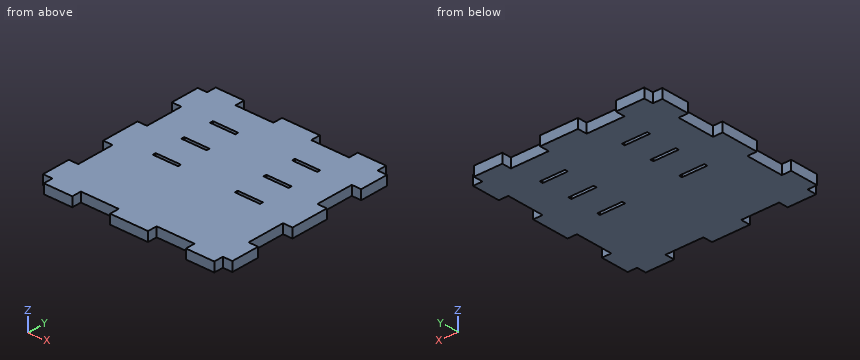
```python
from build123d import *

# Parameters (mm, degrees)
SKETCH1_W           = 190.5
SKETCH1_H           = 190.5
BOSS_EXTRUDE2_DEPTH = 9.525
SKETCH2_W           = 38.1
SKETCH2_H           = 9.525
CUT_EXTRUDE1_DEPTH  = 9.525
SKETCH3_W           = 38.1
SKETCH3_H           = 9.525
CUT_EXTRUDE2_DEPTH  = 9.525
SKETCH4_W           = 9.525
SKETCH4_H           = 38.1
CUT_EXTRUDE3_DEPTH  = 9.525
SKETCH5_W           = 9.525
SKETCH5_H           = 38.1
CUT_EXTRUDE4_DEPTH  = 9.525
SKETCH6_W           = 38.1
SKETCH6_H           = 9.525
CUT_EXTRUDE5_DEPTH  = 9.525
SKETCH7_W           = 38.1
SKETCH7_H           = 9.525
CUT_EXTRUDE6_DEPTH  = 9.525
SKETCH8_W           = 9.525
SKETCH8_H           = 38.1
CUT_EXTRUDE7_DEPTH  = 9.525
SKETCH9_W           = 9.525
SKETCH9_H           = 38.1
CUT_EXTRUDE8_DEPTH  = 9.525
SKETCH10_W          = 9.525
SKETCH10_H          = 9.525
CUT_EXTRUDE9_DEPTH  = 9.525
SKETCH11_W          = 9.525
SKETCH11_H          = 9.525
CUT_EXTRUDE10_DEPTH = 9.525
SKETCH12_W          = 9.525
SKETCH12_H          = 9.525
CUT_EXTRUDE11_DEPTH = 9.525
SKETCH13_W          = 9.525
SKETCH13_H          = 9.525
CUT_EXTRUDE12_DEPTH = 9.525
SKETCH14_W          = 25.4
SKETCH14_H          = 3.175
CUT_EXTRUDE13_DEPTH = 204.230898008


with BuildPart() as part:
    # Sketch1 → Boss-Extrude2 (new body)
    with BuildSketch(Plane.XY):
        with Locations((26.090217391, -67.50326087)):
            Rectangle(SKETCH1_W, SKETCH1_H)
    extrude(amount=BOSS_EXTRUDE2_DEPTH)

    # Sketch2 → Cut-Extrude1 (cut)
    with BuildSketch(Plane.XY.offset(9.525)):
        with Locations((-12.009782609, 22.98423913)):
            Rectangle(SKETCH2_W, SKETCH2_H)
    extrude(amount=-CUT_EXTRUDE1_DEPTH, mode=Mode.SUBTRACT)

    # Sketch3 → Cut-Extrude2 (cut)
    with BuildSketch(Plane.XY.offset(9.525)):
        with Locations((64.190217391, 22.98423913)):
            Rectangle(SKETCH3_W, SKETCH3_H)
    extrude(amount=-CUT_EXTRUDE2_DEPTH, mode=Mode.SUBTRACT)

    # Sketch4 → Cut-Extrude3 (cut)
    with BuildSketch(Plane.XY.offset(9.525)):
        with Locations((116.577717391, -29.40326087)):
            Rectangle(SKETCH4_W, SKETCH4_H)
    extrude(amount=-CUT_EXTRUDE3_DEPTH, mode=Mode.SUBTRACT)

    # Sketch5 → Cut-Extrude4 (cut)
    with BuildSketch(Plane.XY.offset(9.525)):
        with Locations((116.577717391, -105.60326087)):
            Rectangle(SKETCH5_W, SKETCH5_H)
    extrude(amount=-CUT_EXTRUDE4_DEPTH, mode=Mode.SUBTRACT)

    # Sketch6 → Cut-Extrude5 (cut)
    with BuildSketch(Plane.XY.offset(9.525)):
        with Locations((64.190217391, -157.99076087)):
            Rectangle(SKETCH6_W, SKETCH6_H)
    extrude(amount=-CUT_EXTRUDE5_DEPTH, mode=Mode.SUBTRACT)

    # Sketch7 → Cut-Extrude6 (cut)
    with BuildSketch(Plane.XY.offset(9.525)):
        with Locations((-12.009782609, -157.99076087)):
            Rectangle(SKETCH7_W, SKETCH7_H)
    extrude(amount=-CUT_EXTRUDE6_DEPTH, mode=Mode.SUBTRACT)

    # Sketch8 → Cut-Extrude7 (cut)
    with BuildSketch(Plane.XY.offset(9.525)):
        with Locations((-64.397282609, -105.60326087)):
            Rectangle(SKETCH8_W, SKETCH8_H)
    extrude(amount=-CUT_EXTRUDE7_DEPTH, mode=Mode.SUBTRACT)

    # Sketch9 → Cut-Extrude8 (cut)
    with BuildSketch(Plane.XY.offset(9.525)):
        with Locations((-64.397282609, -29.40326087)):
            Rectangle(SKETCH9_W, SKETCH9_H)
    extrude(amount=-CUT_EXTRUDE8_DEPTH, mode=Mode.SUBTRACT)

    # Sketch10 → Cut-Extrude9 (cut)
    with BuildSketch(Plane.XY.offset(9.525)):
        with Locations((-64.397282609, -157.99076087)):
            Rectangle(SKETCH10_W, SKETCH10_H)
    extrude(amount=-CUT_EXTRUDE9_DEPTH, mode=Mode.SUBTRACT)

    # Sketch11 → Cut-Extrude10 (cut)
    with BuildSketch(Plane.XY.offset(9.525)):
        with Locations((-64.397282609, 22.98423913)):
            Rectangle(SKETCH11_W, SKETCH11_H)
    extrude(amount=-CUT_EXTRUDE10_DEPTH, mode=Mode.SUBTRACT)

    # Sketch12 → Cut-Extrude11 (cut)
    with BuildSketch(Plane.XY.offset(9.525)):
        with Locations((116.577717391, 22.98423913)):
            Rectangle(SKETCH12_W, SKETCH12_H)
    extrude(amount=-CUT_EXTRUDE11_DEPTH, mode=Mode.SUBTRACT)

    # Sketch13 → Cut-Extrude12 (cut)
    with BuildSketch(Plane.XY.offset(9.525)):
        with Locations((116.577717391, -157.99076087)):
            Rectangle(SKETCH13_W, SKETCH13_H)
    extrude(amount=-CUT_EXTRUDE12_DEPTH, mode=Mode.SUBTRACT)

    # Sketch14 → Cut-Extrude13 (cut, through all)
    with BuildSketch(Plane.XY.offset(9.525)):
        with Locations((67.365217391, -11.94076087)):
            Rectangle(SKETCH14_W, SKETCH14_H)
        with Locations((-15.184782609, -11.94076087)):
            Rectangle(SKETCH14_W, SKETCH14_H)
        with Locations((67.365217391, -43.69076087)):
            Rectangle(SKETCH14_W, SKETCH14_H)
        with Locations((-15.184782609, -43.69076087)):
            Rectangle(SKETCH14_W, SKETCH14_H)
        with Locations((67.365217391, -75.44076087)):
            Rectangle(SKETCH14_W, SKETCH14_H)
        with Locations((-15.184782609, -75.44076087)):
            Rectangle(SKETCH14_W, SKETCH14_H)
    extrude(amount=-CUT_EXTRUDE13_DEPTH, mode=Mode.SUBTRACT)


solid = part.part
```
Read the model definition and answer for the solid it produces. Units are mm, in the model's axes. Round coordinates to 2 decimals unless told otherwise and drop trailing zeros. Write each loop counter-clockwise with the first axis right and the second up, starting at its lowest first coordinate (ties: lowest second). Pieces come first, ordered by that corner, then holes. Notation, with made-up numbers: (-14.5, 0) - (34.5, 0) arc R13 ccw to (34.5, 19) - close; hole circle Ø1 at (17, -22). An arc over 180 degrees is marked (long way). Use CSV: the item, a comma, the result in double quotes.
Q1. Find section A-A, the plane x = 52. Write down the section's boundary in (y, z) (3 decimals).
Values:
outline,"(-153.228, 0) - (18.222, 0) - (18.222, 9.525) - (-153.228, 9.525) - close"
Q2. Each of these flat-tipped pins is pushed along its axis until it touches: pin 1 Ø5 at (y, z) = (-156.5, 3.5) entering from +X; pin 2 Ø3 at (x, z) = (71, 8) entering from +Y; pin 3 Ø1.6 at (y, z) = (-12.5, 4.5) entering from -X. Where does it stop, or does it pass through?
Values:
pin 1,"stops at x = 111.82"
pin 2,"stops at y = 18.22"
pin 3,"stops at x = -59.63"
Q3. Find section C-C, the plane y = -20.5. Write down the section's boundary in (x, z) (3 decimals).
Values:
outline,"(-59.635, 0) - (111.815, 0) - (111.815, 9.525) - (-59.635, 9.525) - close"
Q4. Find section B-B, the plane z = 4.5. Count the separate pieces of the cut face and the enclosed holes in it, then the cut area to 3 significant figures.
Values:
separate pieces,"1"
enclosed holes,"6"
area,"32,500 mm²"
Q5. Straight lines are drawn through the part: line 1 along Y through (x, z) = (62.5, 1.75); line 2 along Y through (x, z) = (-1, 7.25); line 3 along X through (y, z) = (-28.5, 2). For each, find the intervals that lie inside material, in ascending order.
Values:
line 1,"y = -153.23 to -77.03, -73.85 to -45.28, -42.1 to -13.53, -10.35 to 18.22"
line 2,"y = -153.23 to 18.22"
line 3,"x = -59.63 to 111.82"
